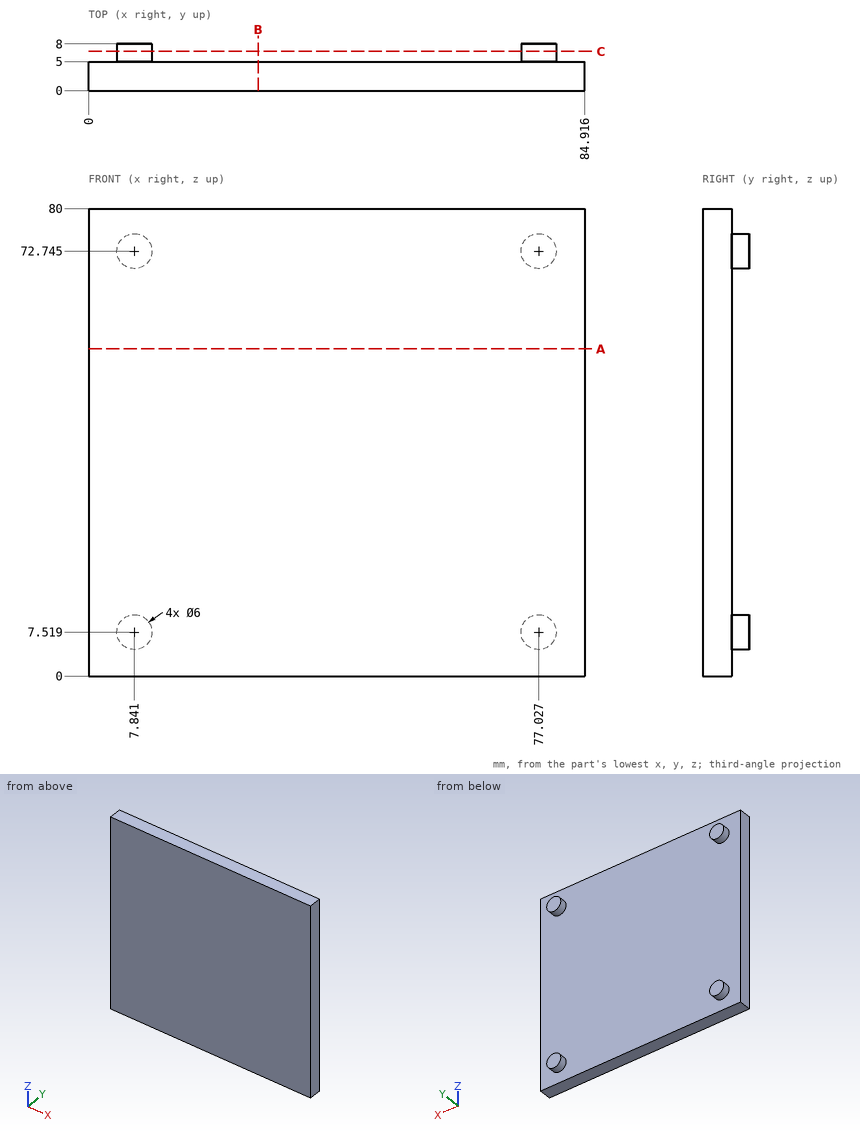
The drawing under review shows one solid part. Ordinate dimensions are in mm from its lowest x, y, z. Coordinates: 2 decimals unless noted, no trailing zeros. Loops run counter-clockwise (first coordinate to the right, second up) from the corner with the lowest first, then second, coordinate; pieces in that order, holes last. Notation, with made-up numbers: (45, 8.25) -> (64, 8.25) arc R25 cw to (64, 36.25) -> close; hole circle Ø2 at (-11.5, -0.75). An arc over 180 degrees is marked (long way). Answer as a JSON object with one key per item and string values.
Q1. Take a section at A-A on z = 56. Give the boundary of the cut face in (x, y).
Answer block:
{"outline": "(0, 0) -> (84.92, 0) -> (84.92, 5) -> (0, 5) -> close"}
Q2. Take a section at C-C on y = 6.75. Give the boundary of the cut face in (x, z) (1 decimal), plus the area to 3 significant figures.
Answer block:
{"outline": "circle Ø6 at (7.8, 7.5); circle Ø6 at (7.8, 72.7); circle Ø6 at (77, 7.5); circle Ø6 at (77, 72.7)", "area": "113 mm^2"}
Q3. To check wall thickness, follow L1, parallel to Y at x = 56.5, z = 28.5. State the ranges of the line that lie inside material, in increasing order.
Answer block:
{"L1": "y = 0 to 5"}
Q4. Take a section at B-B on x = 29. Give the boundary of the cut face in (y, z).
Answer block:
{"outline": "(0, 0) -> (5, 0) -> (5, 80) -> (0, 80) -> close"}
